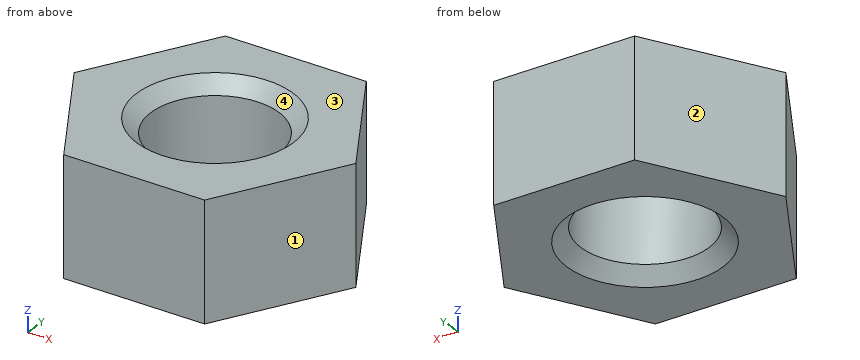
from build123d import *

# Parameters (mm, degrees)
SKETCH1_R           = 3.4
BOSS_EXTRUDE1_DEPTH = 6.3
CHAMFER1_SIZE       = 0.75


with BuildPart() as part:
    # Sketch1 → Boss-Extrude1 (new body)
    with BuildSketch(Plane.XY):
        Polygon((7.505553499, 0), (3.75277675, 6.5), (-3.75277675, 6.5), (-7.505553499, 0), (-3.75277675, -6.5), (3.75277675, -6.5), align=None)
        Circle(SKETCH1_R, mode=Mode.SUBTRACT)
    extrude(amount=BOSS_EXTRUDE1_DEPTH)

    # Chamfer1
    chamfer1_edges = [part.edges().sort_by_distance(p)[0] for p in [
        (-3.4, 0, 0),
        (-3.4, 0, 6.3),
    ]]
    chamfer(chamfer1_edges, length=CHAMFER1_SIZE)


solid = part.part
The model under review builds one solid part; all positions refer to its coordinate system, in mm. Face numbers are marked on the shaded views. Round coordinates to 2 decimals unless told otherwise and drop trailing zeros. Loops run counter-clockwise (first coordinate to the right, second up) from the corner with the lowest first, then second, coordinate; pieces in that order, holes last. Notation, with made-up numbers: M 42.5,38 L 53.5,38 A8 ccw 53.5,42 Z; hole C 32,17.5 d1. An arc over 180 degrees is marked long. Answer as CSV lines item,"result". Start each with the question number.
Item 1: Consider section D-D (x = 4.5). Write out the cut boundary in (y, z).
Item 2: Consider section A-A (x = 0). Write out the cut boundary in (y, z).
Item 3: Consider section C-C (y = -5). Write out the cut boundary in (x, z).
Item 4: Mouldability with a two-part tool opening along Y and no side actions: class the marked faces 1, 2, 3 and 4 as released by +Y, released by -Y, zero draft, split by the parting line, or undercut.
Item 5: Wall thickness on line 1 (Y direction, x = 0, z = 4.5); line 2 (X direction, y = -2.25, z = 1.5); line 3 (X direction, y = 1, z = 5.5): over which ranges is each line inside the solid? List them lowest first. Write a range as [from, to].
Item 6: Consider section B-B (z = 1). Write out the cut boundary in (x, y), then the cut area to 3 significant figures.
Item 7: Insertion check: P1, Ø3, axis at y = 4, z = 2, coming from the +X side. The pin has a flat end and moves straight along its axis. Give the tip position at first contact, or say it passes through.
Answer:
1,outline,"M -5.21,0 L 5.21,0 L 5.21,6.3 L -5.21,6.3 Z"
2,outline,"M -6.5,0 L -4.15,0 L -3.4,0.75 L -3.4,5.55 L -4.15,6.3 L -6.5,6.3 Z; M 3.4,0.75 L 4.15,0 L 6.5,0 L 6.5,6.3 L 4.15,6.3 L 3.4,5.55 Z"
3,outline,"M -4.62,0 L 4.62,0 L 4.62,6.3 L -4.62,6.3 Z"
4,face 1,"released by -Y"
4,face 2,"released by +Y"
4,face 3,"zero draft"
4,face 4,"undercut"
5,line 1,"y = [-6.5, -3.4], [3.4, 6.5]"
5,line 2,"x = [-6.21, -2.55], [2.55, 6.21]"
5,line 3,"x = [-6.93, -3.25], [3.25, 6.93]"
6,outline,"M -7.51,0 L -3.75,-6.5 L 3.75,-6.5 L 7.51,0 L 3.75,6.5 L -3.75,6.5 Z; hole C 0,0 d6.8"
6,area,"110 mm^2"
7,P1,"stops at x = 6.06"
